Source: CAD feature listing. Evaluate the final solid. Frame: model axes, mm. A direction names the side the tool comes from. Round coordinates to 2 decimals unless told otherwise and drop trailing zeros. Write each loop counter-clockwise with the first axis right and the second up, starting at its lowest first coordinate (ties: lowest second). Pieces come first, ordered by that corner, then holes.
from build123d import *

# Parameters (mm, degrees)
SKETCH1_R                = 60
SKETCH1_R_2              = 30
BOSS_EXTRUDE1_DEPTH      = 10
SKETCH2_W                = 10
SKETCH2_H                = 20
BOSS_EXTRUDE2_START      = -20
BOSS_EXTRUDE2_DEPTH      = 20
FILLET1_R                = 2.5
FILLET2_R                = 1
CIRPATTERN1_COUNT        = 6
FILLET1_OF_CIRPATTERN1_R = 2.5
FILLET2_OF_CIRPATTERN1_R = 1
FILLET3_R                = 2


with BuildPart() as part:
    # Sketch1 → Boss-Extrude1 (new, symmetric)
    with BuildSketch(Plane.XY):
        Circle(SKETCH1_R)
        Circle(SKETCH1_R_2, mode=Mode.SUBTRACT)
    extrude(amount=BOSS_EXTRUDE1_DEPTH, both=True)

    # Sketch2 → Cut-Revolve1 (revolve, cut)
    with BuildSketch(Plane(origin=(0, 0, 0), x_dir=(0, 0, -1), z_dir=(1, 0, 0)), mode=Mode.PRIVATE) as cut_revolve1_sk:
        with Locations((0, 60)):
            Rectangle(SKETCH2_W, SKETCH2_H)
    revolve(cut_revolve1_sk.sketch.rotate(Axis((0, 0, 1000), (0, 0, -1)), 90), axis=Axis((0, 0, 1000), (0, 0, -1)), mode=Mode.SUBTRACT)

    # Sketch3 → Boss-Extrude2 (add)
    with BuildSketch(Plane.XY.offset(10).offset(BOSS_EXTRUDE2_START)):
        with BuildLine():
            Line((5.20944533, 29.54423259), (4.341204442, 24.620193825))
            ThreePointArc((4.341204442, 24.620193825), (0, 25), (-4.341204442, 24.620193825))
            Line((-4.341204442, 24.620193825), (-5.20944533, 29.54423259))
            ThreePointArc((-5.20944533, 29.54423259), (0, 30), (5.20944533, 29.54423259))
        make_face()
    boss_extrude2 = extrude(amount=BOSS_EXTRUDE2_DEPTH)

    # Fillet1
    fillet1_edges = [part.edges().sort_by_distance(p)[0] for p in [
        (4.341204442, 24.620193825, 0),
        (-4.341204442, 24.620193825, 0),
    ]]
    fillet(fillet1_edges, radius=FILLET1_R)

    # Fillet2
    fillet2_edges = [part.edges().sort_by_distance(p)[0] for p in [
        (-5.20944533, 29.54423259, 0),
        (5.20944533, 29.54423259, 0),
    ]]
    fillet(fillet2_edges, radius=FILLET2_R)

    # CirPattern1: Boss-Extrude2 ×6 about axis
    cirpattern1_axis = Axis((0, 0, 0), (0, 0, 1))
    for i in range(1, CIRPATTERN1_COUNT):
        add(boss_extrude2.rotate(cirpattern1_axis, i * 360 / CIRPATTERN1_COUNT))

    # Fillet1 of CirPattern1
    fillet1_of_cirpattern1_edges = [part.edges().sort_by_distance(p)[0] for p in [
        (-19.151111078, 16.069690242, 0),
        (-23.49231552, 8.550503583, 0),
        (-23.49231552, -8.550503583, 0),
        (-19.151111078, -16.069690242, 0),
        (-4.341204442, -24.620193825, 0),
        (4.341204442, -24.620193825, 0),
        (19.151111078, -16.069690242, 0),
        (23.49231552, -8.550503583, 0),
        (23.49231552, 8.550503583, 0),
        (19.151111078, 16.069690242, 0),
    ]]
    fillet(fillet1_of_cirpattern1_edges, radius=FILLET1_OF_CIRPATTERN1_R)

    # Fillet2 of CirPattern1
    fillet2_of_cirpattern1_edges = [part.edges().sort_by_distance(p)[0] for p in [
        (-28.190778624, 10.2606043, 0),
        (-22.981333294, 19.283628291, 0),
        (-22.981333294, -19.283628291, 0),
        (-28.190778624, -10.2606043, 0),
        (5.20944533, -29.54423259, 0),
        (-5.20944533, -29.54423259, 0),
        (28.190778624, -10.2606043, 0),
        (22.981333294, -19.283628291, 0),
        (22.981333294, 19.283628291, 0),
        (28.190778624, 10.2606043, 0),
    ]]
    fillet(fillet2_of_cirpattern1_edges, radius=FILLET2_OF_CIRPATTERN1_R)

    # Fillet3
    fillet3_edges = [part.edges().sort_by_distance(p)[0] for p in [
        (-50, 0, -5),
        (-50, 0, 5),
    ]]
    fillet(fillet3_edges, radius=FILLET3_R)


solid = part.part
1) Section query B-B on y = 0. Return the cut outline in (x, z), then the cut area to 3 significant figures.
Taken from the geometry:
outline: (-60, -10) - (-30, -10) - (-30, 10) - (-60, 10) - (-60, 5) - (-52, 5) arc R2 cw to (-50, 3) - (-50, -3) arc R2 cw to (-52, -5) - (-60, -5) - close; (30, -10) - (60, -10) - (60, -5) - (52, -5) arc R2 cw to (50, -3) - (50, 3) arc R2 cw to (52, 5) - (60, 5) - (60, 10) - (30, 10) - close
area: 1,000 mm2
2) Contact query for flat-ended pins moving along their axis: P1, Ø1, axis at x = -12.5, z = 7, coming from the +Y side; P2, Ø10, axis at y = -13, z = 0.5, coming from the -X side; P3, Ø10, axis at y = -15, z = 3, coming from the +X side. Output: stop coordinate, or through.
Taken from the geometry:
P1: stops at y = 58.79
P2: stops at x = -59.02
P3: stops at x = 59.09
3) Pull-direction query (Y, two-part tool) for faces 1 (the face through (-23.951, 9.395, 0.14)), 2 (the face through (47.69, -15.02, -0.04)), 3 (the face through (-1, -26, -10)); classes: released by +Y, released by -Y, zero draft, split by the parting line, or undercut.
Taken from the geometry:
face 1: undercut
face 2: split by the parting line
face 3: zero draft
4) Section query A-A on x = 0. Return the cut outline in (y, z), then the cut area to 3 significant figures.
Taken from the geometry:
outline: (-60, -10) - (-25, -10) - (-25, 10) - (-60, 10) - (-60, 5) - (-52, 5) arc R2 cw to (-50, 3) - (-50, -3) arc R2 cw to (-52, -5) - (-60, -5) - close; (25, -10) - (60, -10) - (60, -5) - (52, -5) arc R2 cw to (50, -3) - (50, 3) arc R2 cw to (52, 5) - (60, 5) - (60, 10) - (25, 10) - close
area: 1,200 mm2
5) Reachability of faces 4 (the face through (3.84, -25.44, 0.14)), 5 (the face through (18, -49, -5)) from +Z, -Z, +X, -X, +Y, -Y: full face, straight path, thin tool, end or side. Return the list, or none.
Taken from the geometry:
face 4: +Z, -Z
face 5: none
6) Material intervals for line 1 (Z direction, x = 52, y = 8); line 2 (Y direction, x = -22, z = 3.5); line 3 (Y direction, x = -20, z = 3.25), sorted ascending.
Taken from the geometry:
line 1: z = -10 to -5, 5 to 10
line 2: y = -44.97 to -20.4, -18.46 to -11.87, 11.87 to 18.46, 20.4 to 44.97
line 3: y = -45.84 to -22.36, 22.36 to 45.84
